from build123d import *

# Parameters (mm, degrees)
BOSS_EXTRUDE1_DEPTH = 30.5
SKETCH2_R           = 3.075
BOSS_EXTRUDE2_DEPTH = 1.6
SKETCH3_R           = 1
BOSS_EXTRUDE3_DEPTH = 6.85
SKETCH4_R           = 4
BOSS_EXTRUDE4_DEPTH = 2
SKETCH5_R           = 1
BOSS_EXTRUDE5_DEPTH = 1.05


with BuildPart() as part:
    # Sketch1 → Boss-Extrude1 (new body)
    with BuildSketch(Plane.XY):
        with BuildLine():
            Line((-7.917543811, 9.15), (7.917543811, 9.15))
            ThreePointArc((7.917543811, 9.15), (12.1, 0), (7.917543811, -9.15))
            Line((7.917543811, -9.15), (-7.917543811, -9.15))
            ThreePointArc((-7.917543811, -9.15), (-12.1, 0), (-7.917543811, 9.15))
        make_face()
    extrude(amount=BOSS_EXTRUDE1_DEPTH)

    # Sketch2 → Boss-Extrude2 (add)
    with BuildSketch(Plane(origin=(0, 0, 0), x_dir=(-1, 0, 0), z_dir=(0, 0, -1))):
        Circle(SKETCH2_R)
    extrude(amount=BOSS_EXTRUDE2_DEPTH)

    # Sketch3 → Boss-Extrude3 (add)
    with BuildSketch(Plane(origin=(0, 0, -1.6), x_dir=(-1, 0, 0), z_dir=(0, 0, -1))):
        Circle(SKETCH3_R)
    extrude(amount=BOSS_EXTRUDE3_DEPTH)

    # Sketch4 → Boss-Extrude4 (add)
    with BuildSketch(Plane.XY.offset(30.5)):
        Circle(SKETCH4_R)
    extrude(amount=BOSS_EXTRUDE4_DEPTH)

    # Sketch5 → Boss-Extrude5 (add)
    with BuildSketch(Plane.XY.offset(32.5)):
        Circle(SKETCH5_R)
    extrude(amount=BOSS_EXTRUDE5_DEPTH)


solid = part.part
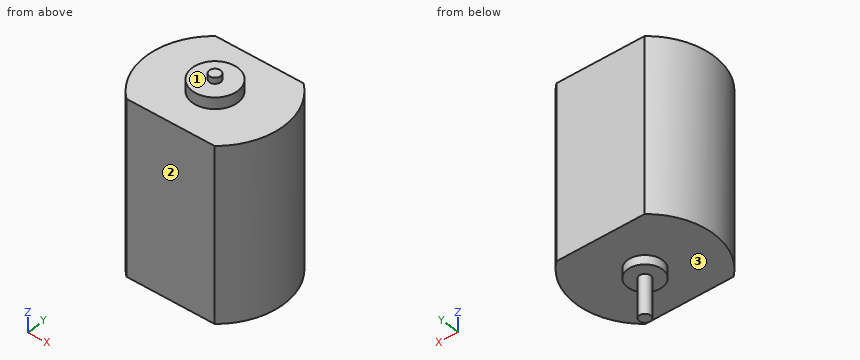
For this review, take the finished solid that the model builds, in its own axes (mm). Face numbers are marked on the shaded views. A direction names the side the tool comes from. Round coordinates to 2 decimals unless told otherwise and drop trailing zeros. Loops run counter-clockwise (first coordinate to the right, second up) from the corner with the lowest first, then second, coordinate; pieces in that order, holes last. Notation, with made-up numbers: (71, 70.5) - (82, 70.5) arc R16 cw to (82, 86.5) - close; hole circle Ø7 at (-9, 21.5). An arc over 180 degrees is marked (long way). One line per item, written item: value. Start each with the question number.
Item 1: Take a section at B-B (y = 0). Give the boundary of the cut face in (x, z) (3 decimals).
Item 2: For the marked faces 1, 2 and 3, list the 3-axis set-ups (+Z, -Z, +X, -X, +Y, -Y) from which the entire face can be reached by the end or side of a thin tool; tool diameter is ignored.
Item 3: For L1, parallel to Z at x = -3.5, y = -3.75; L2, parallel to Z at x = 2.75, y = 2.5; L3, parallel to X at y = 6, z = 4.5, list the stretches that pass through material, from the lowest coordinate up.
Item 4: Take a section at D-D (y = 2). Give the boundary of the cut face in (x, z), plus the area to 3 significant figures.
Item 5: Take a section at A-A (x = 0). Give the boundary of the cut face in (y, z) (3 decimals), plus the area to 3 significant figures.
Item 6: Take a section at C-C (z = 10). Give the boundary of the cut face in (x, y), plus the area to 3 significant figures.
Item 7: Clearance check with flat-ended pins moving along their axes: pin 1 Ø2.5 at (x, y) = (-1.5, -2) entering from +Z; pin 2 Ø5.5 at (x, y) = (-1.5, 2) entering from -Z; pin 3 Ø3 at (y, z) = (3, 17) entering from -X. State where each tip first meets the part, or that it passes through.
Answer below:
1. outline: (-12.1, 0) - (-3.075, 0) - (-3.075, -1.6) - (-1, -1.6) - (-1, -8.45) - (1, -8.45) - (1, -1.6) - (3.075, -1.6) - (3.075, 0) - (12.1, 0) - (12.1, 30.5) - (4, 30.5) - (4, 32.5) - (1, 32.5) - (1, 33.55) - (-1, 33.55) - (-1, 32.5) - (-4, 32.5) - (-4, 30.5) - (-12.1, 30.5) - close
2. face 1: +Z
2. face 2: +Z, -Z, +X, -X, -Y
2. face 3: -Z
3. L1: z = 0 to 30.5
3. L2: z = 0 to 32.5
3. L3: x = -10.51 to 10.51
4. outline: (-11.93, 0) - (-2.34, 0) - (-2.34, -1.6) - (2.34, -1.6) - (2.34, 0) - (11.93, 0) - (11.93, 30.5) - (3.46, 30.5) - (3.46, 32.5) - (-3.46, 32.5) - (-3.46, 30.5) - (-11.93, 30.5) - close
4. area: 749 mm2
5. outline: (-9.15, 0) - (-3.075, 0) - (-3.075, -1.6) - (-1, -1.6) - (-1, -8.45) - (1, -8.45) - (1, -1.6) - (3.075, -1.6) - (3.075, 0) - (9.15, 0) - (9.15, 30.5) - (4, 30.5) - (4, 32.5) - (1, 32.5) - (1, 33.55) - (-1, 33.55) - (-1, 32.5) - (-4, 32.5) - (-4, 30.5) - (-9.15, 30.5) - close
5. area: 600 mm2
6. outline: (-7.92, -9.15) - (7.92, -9.15) arc R12.1 ccw to (7.92, 9.15) - (-7.92, 9.15) arc R12.1 ccw to start
6. area: 396 mm2
7. pin 1: stops at z = 32.5
7. pin 2: stops at z = -8.45
7. pin 3: stops at x = -12.01
